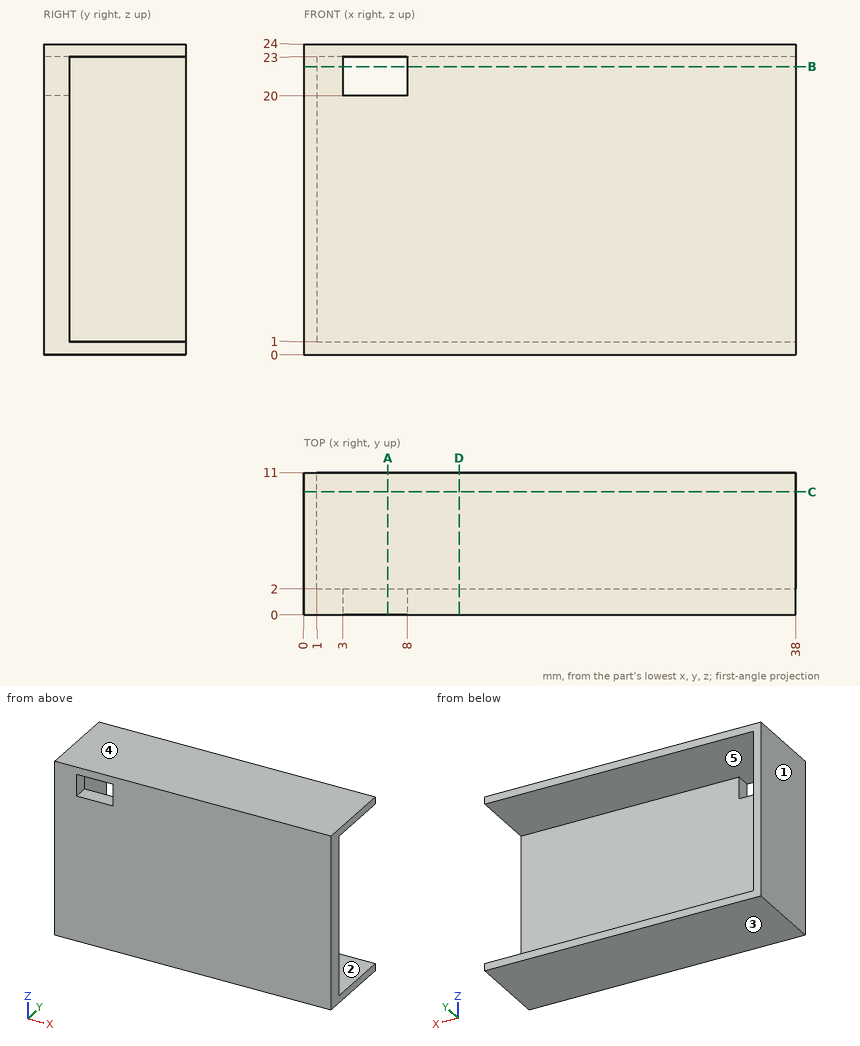
Check sheet for the drawn part. Datum: minimum x, y, z corner. Units: mm. A direction names the side the tool comes from. Coordinates: 2 decimals unless noted, no trailing zeros. Loops run counter-clockwise (first coordinate to the right, second up) from the corner with the lowest first, then second, coordinate; pieces in that order, holes last. Notation, with made-up numbers: (42, -1.75) -> (63, -1.75) arc R22 ccw to (63, 8.25) -> close; hole circle Ø4 at (81, -18). An arc over 180 degrees is marked (long way). Answer in a Markdown table with one row per item.
1) Draft check along Z on the marked faces 3, 4 and 5. Enter one of: released by +Z, released by -Z, zero draft, split by the parting line, or undercut.
The answers:
| item | result |
|---|---|
| face 3 | released by -Z |
| face 4 | released by +Z |
| face 5 | undercut |
2) Section check A-A (x = 6.5). Record the cut outline in (y, z).
The answers:
| item | result |
|---|---|
| outline | (0, 0) -> (11, 0) -> (11, 1) -> (2, 1) -> (2, 20) -> (0, 20) -> close; (0, 23) -> (11, 23) -> (11, 24) -> (0, 24) -> close |
3) Section check D-D (x = 12). Record the cut outline in (y, z), and give its area (3 significant figures).
The answers:
| item | result |
|---|---|
| outline | (0, 0) -> (11, 0) -> (11, 1) -> (2, 1) -> (2, 23) -> (11, 23) -> (11, 24) -> (0, 24) -> close |
| area | 66.0 mm2 |
4) Depth check by flat-ended pin: P1, Ø12, axis at x = 28.5, z = 11, coming from the +Y side; P2, Ø3, axis at y = 6.5, z = 3.5, coming from the +X side. Enter the tip coordinate at first touch or a pass-through.
The answers:
| item | result |
|---|---|
| P1 | stops at y = 2 |
| P2 | stops at x = 1 |
5) Access from +Z, -Z, +X, -X, +Y, -Y to the whole of each face (thin tool, end or side, straight path). Record for the marked faces 1 and 2.
The answers:
| item | result |
|---|---|
| face 1 | +Z, -Z, -X, +Y, -Y |
| face 2 | +X, +Y |
6) Scan lines: line 1 along Z through (x, y) = (33, 3.5); line 2 along Z through (x, y) = (5, 1.75); line 3 along Y through (x, z) = (13.5, 9.5). Record each from-to range of solid material in increasing order. Write a range as from..to.
The answers:
| item | result |
|---|---|
| line 1 | z = 0..1, 23..24 |
| line 2 | z = 0..20, 23..24 |
| line 3 | y = 0..2 |
7) Section check C-C (y = 9.5). Record the cut outline in (x, z), and give its area (3 significant figures).
The answers:
| item | result |
|---|---|
| outline | (0, 0) -> (38, 0) -> (38, 1) -> (1, 1) -> (1, 23) -> (38, 23) -> (38, 24) -> (0, 24) -> close |
| area | 98.0 mm2 |
8) Section check B-B (z = 22.25). Record the cut outline in (x, y), and give its area (3 significant figures).
The answers:
| item | result |
|---|---|
| outline | (0, 0) -> (3, 0) -> (3, 2) -> (1, 2) -> (1, 11) -> (0, 11) -> close; (8, 0) -> (38, 0) -> (38, 2) -> (8, 2) -> close |
| area | 75.0 mm2 |
